Could you check a few things on this model? Use its own coordinates, in mm. Face numbers are marked on the shaded views. A direction names the side the tool comes from. Coordinates: 2 decimals unless noted, no trailing zeros. Loops run counter-clockwise (first coordinate to the right, second up) from the corner with the lowest first, then second, coordinate; pieces in that order, holes last. Notation, with made-up numbers: (-14, 12) -> (1, 12) arc R23 ccw to (1, 37) -> close; hole circle Ø2 at (-14, -5.5). An arc over 180 degrees is marked (long way). One line per question, with ' | ' between items.
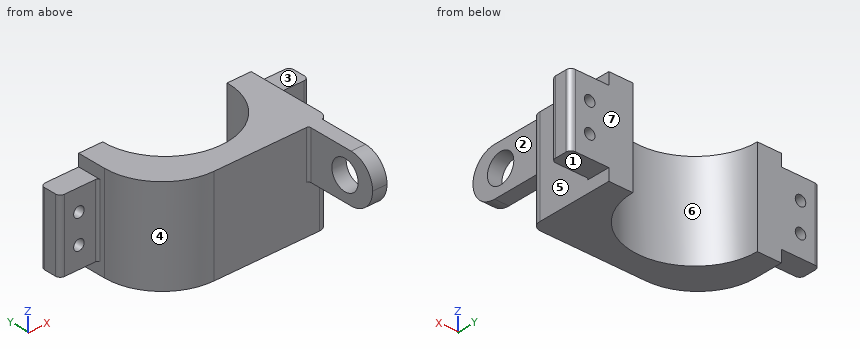
Autodesk Fusion 360 part; units mm, degrees
sketch "Sketch1" plane through (0, 0, 0) normal (0, 0, 1) x (1, 0, 0)
  line L0 (0, 0) -> (36, 0)
  line L1 (36, 0) -> (36, 18)
  line L2 (36, 18) -> (0, 18)
  line L3 (0, 18) -> (0, 0)
  dimension "d1" = 36
  dimension "d2" = 18
extrude "Extrude1" add sketch "Sketch1" along normal blind 20
sketch "Sketch2" plane through (0, 0, 20) normal (0, 0, 1) x (-1, 0, 0)
  line L0 (0, -18) -> (0, 0)
  line L1 (0, 0) -> (-36, 0)
  line L2 (-36, 0) -> (-36, -18)
  line L3 (-36, -18) -> (0, -18)
  circle A0 centre (-18, -18) radius 13
  dimension "d5" = 26
extrude "Extrude2" cut sketch "Sketch2" against normal blind 20 contours L3 A0 picked at (-19.0768, -11.2377)
ref_plane "WorkPlane1" through (0, 20, 0) normal (0, 1, 0) x (0, 0, 1)
sketch "Sketch7" plane through (0, 0, 0) normal (0, -1, 0) x (1, 0, 0)
  line L0 (0, 0) -> (36, 0)
  line L1 (36, 20) -> (0, 20)
  line L2 (0, 20) -> (0, 0)
  line L3 (18, 10) -> (18, 23) construction
  line L4 (36, 0) -> (36, 20)
sketch "Sketch6" plane through (36, 0, 0) normal (1, 0, 0) x (0, 1, 0)
  line L0 (0, 0) -> (18, 0)
  line L1 (18, 0) -> (18, 20)
  line L2 (18, 20) -> (0, 20)
  line L3 (0, 20) -> (0, 0)
  line L4 (0, 20) -> (18, 0) construction
  line L5 (0, 0) -> (18, 20) construction
  line L6 (9, 10) -> (18, 10) construction
  line L7 (9, 10) -> (9, 0) construction
  line L8 (9, 10) -> (9, 20) construction
  line L9 (13.5, 17.5) -> (18, 17.5) construction
  line L10 (13.5, 5) -> (13.5, 10) construction
  line L11 (18, 7.5) -> (18, 12.5311)
  line L12 (13.5, 17.5) -> (18, 17.5)
  line L13 (18, 17.5) -> (18, 2.5)
  line L14 (18, 2.5) -> (13.5, 2.5)
  line L15 (13.5, 2.5) -> (13.5, 17.5)
  dimension "d25" = 15
  dimension "d26" = 4.5
  dimension "d34" = 7.5
extrude "Extrude7" add sketch "Sketch6" along normal blind 8 contours L1 L11 L12 L13 L14 L15
sketch "Sketch11" plane through (0, 13.5, 0) normal (0, -1, 0) x (1, 0, 0)
  line L0 (36, 17.5) -> (36, 2.5)
  line L1 (36, 2.5) -> (44, 2.5)
  line L2 (44, 2.5) -> (44, 17.5)
  line L3 (44, 17.5) -> (36, 17.5)
  circle A0 centre (40, 13) radius 1.1
  circle A1 centre (40, 7) radius 1.1
  line L4 (36, 0) -> (36, 20)
  line L5 (36, 20) -> (0, 20)
  line L6 (18, 10) -> (18, 23)
  circle A2 centre (-4, 13) radius 1.1
  circle A3 centre (-4, 7) radius 1.1
  dimension "d30" = 2.2
  dimension "d31" = 2.2
  dimension "d35" = 6
  dimension "d36" = 4
  dimension "d37" = 4
  dimension "d38" = 7
sketch "Sketch12" plane through (0, 0, 0) normal (-1, 0, 0) x (0, -1, 0)
  line L0 (-18, 0) -> (0, 0)
  line L1 (0, 0) -> (0, 20)
  line L2 (0, 20) -> (-18, 20)
  line L3 (-18, 20) -> (-18, 0)
  line L4 (-18, 17.5) -> (-13.5, 17.5)
  line L5 (-13.5, 17.5) -> (-13.5, 2.5)
  line L6 (-13.5, 2.5) -> (-18, 2.5)
  line L7 (-18, 2.5) -> (-18, 17.5)
  line L8 (-18, 10) -> (-8, 10) construction
  dimension "d39" = 15
  dimension "d40" = 7.5
  dimension "d41" = 4.5
extrude "Extrude8" add sketch "Sketch12" along normal blind 8 contours L3 L4 L5 L6 L7
extrude "Extrude9" cut sketch "Sketch11" against normal blind 4.5 contours A0 | A1 | A2 | A3
sketch "Sketch13" plane through (0, 0, 20) normal (0, 0, 1) x (-1, 0, 0)
  arc A0 (-5, -18) -> (-31, -18) centre (-18, -18) ccw
  line L0 (-5, -18) -> (0, -18)
  line L1 (0, -18) -> (0, 0)
  line L2 (0, 0) -> (-36, 0)
  line L3 (-36, 0) -> (-36, -18)
  line L4 (-36, -18) -> (-31, -18)
  line L5 (-34.8, -18) -> (-34.8, 0) construction
  dimension "d46" = 3.8
sketch "Sketch14" plane through (18, 0, 10) normal (0, -1, 0) x (1, 0, 0)
  line L0 (16.8, 10) -> (13.8, 10)
  line L1 (13.8, 10) -> (13.8, 0)
  line L2 (13.8, 0) -> (16.8, 0)
  line L3 (16.8, 0) -> (16.8, 10)
  point P0 (16.8, 10)
  dimension "d47" = 3
  dimension "d48" = 10
extrude "Extrude10" add sketch "Sketch14" along normal blind 14.8
sketch "Sketch15" plane through (34.8, 0, 0) normal (1, 0, 0) x (0, 1, 0)
  line L0 (0, 10) -> (0, 20)
  line L1 (0, 20) -> (-14.8, 20)
  line L2 (-14.8, 20) -> (-14.8, 10)
  line L3 (-14.8, 10) -> (0, 10)
  circle A0 centre (-8.4, 15) radius 3.05
  dimension "d51" = 6.1
  dimension "d52" = 6.4
  dimension "d53" = 5
extrude "Extrude11" cut sketch "Sketch15" against normal blind 3 contours A0
fillet "Fillet1" radius 5 2 edges at (33.3, -14.8, 20) (33.3, -14.8, 10)
fillet "Fillet2" radius 2 1 edges at (36, 0, 10)
fillet "Fillet3" radius 12 1 edges at (0, 0, 10)
fillet "Fillet4" radius 0.5 1 edges at (0, 13.5, 10)
fillet "Fillet5" radius 1 2 edges at (-8, 18, 10) (-8, 13.5, 10)
fillet "Fillet6" radius 1 2 edges at (44, 13.5, 10) (44, 18, 10)
fillet "Fillet7" radius 0.5 1 edges at (36, 13.5, 10)
fillet "Fillet8" radius 0.5 1 edges at (31.8, 0, 15)
Q1. Imagine slicing it at D-D on z = 13. Give the number of separate pieces and of enclosed holes in the cut face, plus the area to 3 significant figures.
Values follow:
separate pieces: 4 | enclosed holes: 0 | area: 432 mm2
Q2. Imagine slicing it at A-A on y = -8.4. Write out the boundary of the cut face in (x, z).
Values follow:
outline: (31.8, 10) -> (34.8, 10) -> (34.8, 11.95) -> (31.8, 11.95) -> close; (31.8, 18.05) -> (34.8, 18.05) -> (34.8, 20) -> (31.8, 20) -> close
Q3. Please list where these lines run through material, in increasing order: L1, parallel to Z at x = -4, y = 15; L2, parallel to Y at x = 39, z = 9.75; L3, parallel to Z at x = 32.75, y = -8.4. Write a range as [from, to].
Values follow:
L1: z = [2.5, 5.9], [8.1, 11.9], [14.1, 17.5] | L2: y = [13.5, 18] | L3: z = [10, 11.95], [18.05, 20]
Q4. Imagine slicing it at C-C on z = 7. Write out the boundary of the cut face in (x, y).
Values follow:
outline: (-8, 14.5) arc R1 ccw to (-7, 13.5) -> (-5.1, 13.5) -> (-5.1, 18) -> (-7, 18) arc R1 ccw to (-8, 17) -> close; (-2.9, 13.5) -> (-0.5, 13.5) arc R0.5 cw to (0, 13) -> (0, 12) arc R12 ccw to (12, 0) -> (34, 0) arc R2 ccw to (36, 2) -> (36, 13) arc R0.5 cw to (36.5, 13.5) -> (38.9, 13.5) -> (38.9, 18) -> (31, 18) arc R13 cw to (5, 18) -> (-2.9, 18) -> close; (41.1, 13.5) -> (43, 13.5) arc R1 ccw to (44, 14.5) -> (44, 17) arc R1 ccw to (43, 18) -> (41.1, 18) -> close
Q5. We'd pull the mould along X, two halves only. Please class the marked faces 4, 5, 6 and 7: released by +X, released by -X, zero draft, split by the parting line, or undercut.
Values follow:
face 4: released by -X | face 5: released by +X | face 6: undercut | face 7: zero draft
Q6. For the marked faces 1, 2 and 3, which set-ups out of +Z, -Z, +X, -X, +Y, -Y let a thin tool reach every point of the face, with its end or its side?
Values follow:
face 1: -Z, +X, +Y, -Y | face 2: +Z, -Z, +X, -Y | face 3: +Z, +X, +Y, -Y
Q7. Imagine slicing it at B-B on x = -4. Write out the boundary of the cut face in (y, z), plus the area to 3 significant figures.
Values follow:
outline: (13.5, 2.5) -> (18, 2.5) -> (18, 5.9) -> (13.5, 5.9) -> close; (13.5, 8.1) -> (18, 8.1) -> (18, 11.9) -> (13.5, 11.9) -> close; (13.5, 14.1) -> (18, 14.1) -> (18, 17.5) -> (13.5, 17.5) -> close | area: 47.7 mm2
Q8. For pin 1 (5.5 mm diameter, centred on x = 41.5, y = 14.5, fed in from -Z); pin 2 (3 mm diameter, centred on x = 3.5, z = 14, fed in from -Y); pin 3 (2 mm diameter, centred on x = 24, z = 10.5, fed in from +Y), each with a flat end and sliding along its axis, tell me the tip position at first contact or that it passes through.
Values follow:
pin 1: stops at z = 2.5 | pin 2: stops at y = 2.25 | pin 3: stops at y = 7.05
